```python
from build123d import *

# Parameters (mm, degrees)
CUT_EXTRUDE1_DEPTH = 18.5
FILLET1_R          = 5


with BuildPart() as part:
    # Sketch2 → Revolve1 (revolve)
    with BuildSketch(Plane.XY):
        Polygon((12.5, 0), (62.5, 0), (62.5, 17.5), (60.5, 17.5), (60.5, 9.5), (59, 9.5), (59, 3), (12.5, 3), align=None)
    revolve(axis=Axis((0, 0, 0), (0, 1, 0)))

    # Sketch3 → Cut-Extrude1 (cut, through all)
    with BuildSketch(Plane.XZ):
        with BuildLine():
            Line((-14.235047481, 53.125920446), (-6.698729811, 25))
            Line((-6.698729811, 25), (6.698729811, 25))
            Line((6.698729811, 25), (14.235047481, 53.125920446))
            ThreePointArc((14.235047481, 53.125920446), (0, 55), (-14.235047481, 53.125920446))
        make_face()
    extrude(amount=-CUT_EXTRUDE1_DEPTH, mode=Mode.SUBTRACT)

    # Fillet1
    fillet1_edges = [part.edges().sort_by_distance(p)[0] for p in [
        (6.698729811, 1.5, 25),
        (-6.698729811, 1.5, 25),
        (-14.235047481, 1.5, 53.125920446),
        (14.235047481, 1.5, 53.125920446),
    ]]
    fillet(fillet1_edges, radius=FILLET1_R)


solid = part.part
```
The model under review builds one solid part; all positions refer to its coordinate system, in mm. A direction names the side the tool comes from. Coordinates: 2 decimals unless noted, no trailing zeros. Order: outer loops, then holes, each group sorted by start corner. A loop starts at its lowest first (then second) coordinate and runs counter-clockwise, first axis right, second up. Notation, with made-up numbers: (89, 42.25) -> (101, 42.25) arc R30 ccw to (101, 72.25) -> close; hole circle Ø1 at (-26, 32.5). An arc over 180 degrees is marked (long way). Answer in a Markdown table with one row per item. Add a question column.
Item 1: We need section D-D on z = -45. Write out the cut boundary in (x, y).
Item 2: We need section C-C on y = 14.25. Write out the cut boundary in (x, z).
Item 3: Machinability: for faces 5 (the cylindrical face through (-12.28, 1.52, 52.01)), 6 (the flat face through (-13, 0, -1)), 7 (the cylindrical face through (56.275, 6.204, -17.722)), which of the approach directions +Z, -Z, +X, -X, +Y, -Y give a long, thin tool a straight path to every point of the face, cutting with its end or side? Answer none if there is none.
Item 4: We need section B-B on z = 0. Write out the cut boundary in (x, y), plus the area to 4 significant figures.
Item 5: Mouldability with a two-part tool opening along Z and no side actions: class faces 1 (the cylindrical face through (5.869, 1.521, 26.006)), 2 (the flat face through (-1, 3, -14)), 3 (the cylindrical face through (-62.44, 8.87, -2.75)), 4 (the flat face through (-33, 17.5, -51)) as +Z half, -Z half, draft (parallel to the pull), parting line (faces both ways), or undercut.
Item 6: To check wall thickness, follow probe 1 along Z at (x, y) = (0, 1.2); probe 2 along Z at (x, y) = (0, 5); probe 3 along Y at (x, z) = (43, -3). State the ranges of each line that lie inside material, in increasing order.
Item 7: We need section A-A on x = 0. Write out the cut boundary in (y, z), plus the area to 4 significant figures.
Item 8: Clearance check with flat-ended pins moving along their axes: pin 1 (0.9 mm diameter, centred on x = -0.5, y = 2, fed in from +Z); pin 2 (3 mm diameter, centred on x = 32, y = 2, fed in from +Z); pin 3 (1.5 mm diameter, centred on y = 13, z = 29.5, fed in from +X). State where each tip first meets the part, or that it passes through.
Final values:
| question | item | result |
|---|---|---|
| 1 | outline | (-43.37, 0) -> (43.37, 0) -> (43.37, 17.5) -> (40.44, 17.5) -> (40.44, 9.5) -> (38.16, 9.5) -> (38.16, 3) -> (-38.16, 3) -> (-38.16, 9.5) -> (-40.44, 9.5) -> (-40.44, 17.5) -> (-43.37, 17.5) -> close |
| 2 | outline | circle Ø125 at (0, 0); hole circle Ø121 at (0, 0) |
| 3 | face 5 | +Y, -Y |
| 3 | face 6 | +Z, -Z, +X, -X, -Y |
| 3 | face 7 | +Y |
| 4 | outline | (-62.5, 0) -> (-12.5, 0) -> (-12.5, 3) -> (-59, 3) -> (-59, 9.5) -> (-60.5, 9.5) -> (-60.5, 17.5) -> (-62.5, 17.5) -> close; (12.5, 0) -> (62.5, 0) -> (62.5, 17.5) -> (60.5, 17.5) -> (60.5, 9.5) -> (59, 9.5) -> (59, 3) -> (12.5, 3) -> close |
| 4 | area | 377.5 mm2 |
| 5 | face 1 | undercut |
| 5 | face 2 | undercut |
| 5 | face 3 | parting line |
| 5 | face 4 | draft |
| 6 | probe 1 | z = -62.5 to -12.5, 12.5 to 25, 55 to 62.5 |
| 6 | probe 2 | z = -62.5 to -59, 59 to 62.5 |
| 6 | probe 3 | y = 0 to 3 |
| 7 | outline | (0, -62.5) -> (17.5, -62.5) -> (17.5, -60.5) -> (9.5, -60.5) -> (9.5, -59) -> (3, -59) -> (3, -12.5) -> (0, -12.5) -> close; (0, 12.5) -> (3, 12.5) -> (3, 25) -> (0, 25) -> close; (0, 55) -> (3, 55) -> (3, 59) -> (9.5, 59) -> (9.5, 60.5) -> (17.5, 60.5) -> (17.5, 62.5) -> (0, 62.5) -> close |
| 7 | area | 287.5 mm2 |
| 8 | pin 1 | stops at z = 62.5 |
| 8 | pin 2 | stops at z = 54.55 |
| 8 | pin 3 | stops at x = 55.49 |
